Answer from the drawing. Dimensions are ordinates in mm from the lowest x, y and z of the part. A direction names the side the tool comes from. Round coordinates to 2 decimals unless told otherwise and drop trailing zeros. Loops run counter-clockwise (first coordinate to the right, second up) from the corner with the lowest first, then second, coordinate; pieces in that order, holes last. Notation, with made-up numbers: (-33, 21.25) -> (26, 21.25) arc R33 ccw to (26, 52.25) -> close; hole circle Ø11 at (41, 60). An arc over 180 degrees is marked (long way). Use CSV: the item, a comma, the result in double quotes. Start each with the question number.
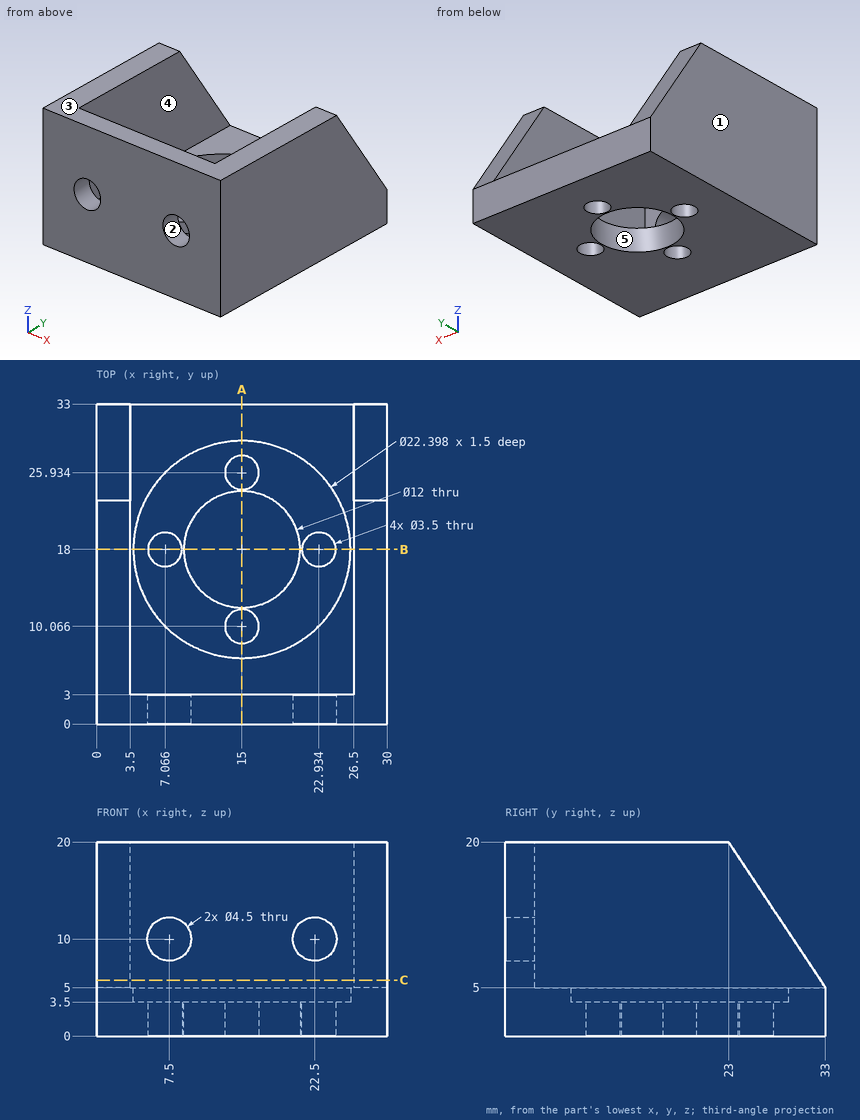
Q1. Which of the six approach directions +Z, -Z, +X, -X, +Y, -Y give full straight-line access (tool end or side, diameter ignored) to the marked faces 4 and 5?
Q2. Section B-B, the plane y = 18 is taken. Write down the section's boundary in (x, z).
Q3. Section A-A, the plane x = 15 is taken. Write down the section's boundary in (y, z).
Q4. Straight lines are drawn through the part: line 1 (X direction, y = 23.5, z = 14); line 2 (Z direction, x = 7.5, y = 1.35); line 3 (Y direction, x = 22.5, z = 17.5). For each, find the intervals that lie inside material, in ascending order. Write a range as from..to.
Q5. For a pull along X with two mould halves and no side action, classify the marked faces 1, 2 and 3 as pulls with the +X half, pulls with the -X half, needs draft (parallel to the pull), parting line crosses it, or undercut.
Q6. Each of these flat-tipped pins is pushed along its axis until it touches: pin 1 (2.5 mm diameter, centred on x = 22.5, z = 10, fed in from +Y); pin 2 (4.5 mm diameter, centred on x = 15, y = 10.07, fed in from +Z). Where does it stop, or does it pass through?
Q7. Section C-C, the plane z = 5.75 is taken. Write down the section's boundary in (x, y).
Report:
1,face 4,"+Z, +Y"
1,face 5,"+Z, -Z"
2,outline,"(0, 0) -> (5.32, 0) -> (5.32, 3.5) -> (3.8, 3.5) -> (3.8, 5) -> (3.5, 5) -> (3.5, 20) -> (0, 20) -> close; (8.82, 0) -> (9, 0) -> (9, 3.5) -> (8.82, 3.5) -> close; (21, 0) -> (21.18, 0) -> (21.18, 3.5) -> (21, 3.5) -> close; (24.68, 0) -> (30, 0) -> (30, 20) -> (26.5, 20) -> (26.5, 5) -> (26.2, 5) -> (26.2, 3.5) -> (24.68, 3.5) -> close"
3,outline,"(0, 0) -> (8.32, 0) -> (8.32, 3.5) -> (6.8, 3.5) -> (6.8, 5) -> (3, 5) -> (3, 20) -> (0, 20) -> close; (11.82, 0) -> (12, 0) -> (12, 3.5) -> (11.82, 3.5) -> close; (24, 0) -> (24.18, 0) -> (24.18, 3.5) -> (24, 3.5) -> close; (27.68, 0) -> (33, 0) -> (33, 5) -> (29.2, 5) -> (29.2, 3.5) -> (27.68, 3.5) -> close"
4,line 1,"x = 0..3.5, 26.5..30"
4,line 2,"z = 0..7.75, 12.25..20"
4,line 3,"y = 0..3"
5,face 1,"pulls with the -X half"
5,face 2,"undercut"
5,face 3,"needs draft"
6,pin 1,"passes through"
6,pin 2,"stops at z = 3.5"
7,outline,"(0, 0) -> (30, 0) -> (30, 32.5) -> (26.5, 32.5) -> (26.5, 3) -> (3.5, 3) -> (3.5, 32.5) -> (0, 32.5) -> close"
